from build123d import *

# Parameters (mm, degrees)
IZIM1_R                     = 7.95
Y_KSEKLIK_EKSTR_ZYON1_DEPTH = 8
IZIM2_R                     = 1.35
KES_EKSTR_ZYON1_DEPTH       = 50
IZIM3_R                     = 1.35
KES_EKSTR_ZYON2_DEPTH       = 29
KES_EKSTR_ZYON3_DEPTH       = 10
Y_KSEKLIK_EKSTR_ZYON2_REACH = 46.587
IZIM5_W                     = 5.529758539
IZIM5_H                     = 16.549351305
IZIM6_R                     = 1.35
KES_EKSTR_ZYON4_DEPTH       = 10
KES_EKSTR_ZYON5_DEPTH       = 2.5
Y_KSEKLIK_EKSTR_ZYON3_DEPTH = 0.5


with BuildPart() as part:
    # Çizim1 → Yükseklik-Ekstrüzyon1 (new body)
    with BuildSketch(Plane.XY):
        with BuildLine():
            Line((0, 0), (32, 0))
            Line((32, 0), (32, 8))
            Line((32, 8), (31.5, 8))
            ThreePointArc((31.5, 8), (28.671572875, 9.171572875), (27.5, 12))
            Line((27.5, 12), (27.5, 18))
            ThreePointArc((27.5, 18), (28.671572875, 20.828427125), (31.5, 22))
            Line((31.5, 22), (32, 22))
            Line((32, 22), (32, 30))
            Line((32, 30), (0, 30))
            Line((0, 30), (0, 22))
            Line((0, 22), (0.5, 22))
            ThreePointArc((0.5, 22), (3.328427125, 20.828427125), (4.5, 18))
            Line((4.5, 18), (4.5, 12))
            ThreePointArc((4.5, 12), (3.328427125, 9.171572875), (0.5, 8))
            Line((0.5, 8), (0, 8))
            Line((0, 8), (0, 0))
        make_face()
        with Locations((16, 15)):
            Circle(IZIM1_R, mode=Mode.SUBTRACT)
    extrude(amount=Y_KSEKLIK_EKSTR_ZYON1_DEPTH)

    # Çizim2 → Kes-Ekstrüzyon1 (cut)
    with BuildSketch(Plane(origin=(32, 0, 0), x_dir=(0, 0, -1), z_dir=(1, 0, 0))):
        with Locations((-4, 4)):
            Circle(IZIM2_R)
        with Locations((-4, 26)):
            Circle(IZIM2_R)
    extrude(amount=-KES_EKSTR_ZYON1_DEPTH, mode=Mode.SUBTRACT)

    # Çizim3 → Kes-Ekstrüzyon2 (cut)
    with BuildSketch(Plane.ZY.offset(-4.5)):
        with Locations(Location((4, 15, 0), (0, 0, 270))):
            Circle(IZIM3_R)
    extrude(amount=-KES_EKSTR_ZYON2_DEPTH, mode=Mode.SUBTRACT)

    # Çizim4 → Kes-Ekstrüzyon3 (cut)
    with BuildSketch(Plane(origin=(0, 0, 0), x_dir=(-1, 0, 0), z_dir=(0, 0, -1))):
        Polygon((-16, 30), (-16, 0), (9.241069926, -10.278514345), (11.843794838, 24.557008953), (11.843794838, 39.531622814), align=None)
    extrude(amount=-KES_EKSTR_ZYON3_DEPTH, mode=Mode.SUBTRACT)

    # Yükseklik-Ekstrüzyon2: up to this face of the body (flat: up to its plane)
    y_kseklik_ekstr_zyon2_end = Plane(part.part.faces().sort_by_distance((24.391799767, 15, 8))[0])
    # Çizim5 → Yükseklik-Ekstrüzyon2 (add, up to the picked face)
    with BuildSketch(Plane(origin=(0, 0, 0), x_dir=(-1, 0, 0), z_dir=(0, 0, -1)), mode=Mode.PRIVATE) as y_kseklik_ekstr_zyon2_sk1:
        with Locations((-29.235120731, 13.725324347)):
            Rectangle(IZIM5_W, IZIM5_H)
    y_kseklik_ekstr_zyon2_tool1 = split(extrude(y_kseklik_ekstr_zyon2_sk1.sketch, amount=-Y_KSEKLIK_EKSTR_ZYON2_REACH, mode=Mode.PRIVATE), bisect_by=y_kseklik_ekstr_zyon2_end, keep=Keep.BOTH, mode=Mode.PRIVATE)
    add(y_kseklik_ekstr_zyon2_tool1.solids().sort_by(Axis((29.235121, 13.725324, 0), (0, 0, 1)))[0])

    # Çizim6 → Kes-Ekstrüzyon4 (cut)
    with BuildSketch(Plane.ZY.offset(-26.470241461)):
        with Locations(Location((4, 15, 0), (0, 0, 270))):
            Circle(IZIM6_R)
    extrude(amount=-KES_EKSTR_ZYON4_DEPTH, mode=Mode.SUBTRACT)

    # Çizim7 → Kes-Ekstrüzyon5 (cut)
    with BuildSketch(Plane(origin=(32, 0, 0), x_dir=(0, 0, -1), z_dir=(1, 0, 0))):
        Polygon((-2.41228676, 28.75), (-5.58771324, 28.75), (-7.175426481, 26), (-5.58771324, 23.25), (-2.41228676, 23.25), (-0.824573519, 26), align=None)
        Polygon((-0.824573519, 15), (-2.41228676, 17.75), (-5.58771324, 17.75), (-7.175426481, 15), (-5.58771324, 12.25), (-2.41228676, 12.25), align=None)
        Polygon((-2.41228676, 6.75), (-5.58771324, 6.75), (-7.175426481, 4), (-5.58771324, 1.25), (-2.41228676, 1.25), (-0.824573519, 4), align=None)
    extrude(amount=-KES_EKSTR_ZYON5_DEPTH, mode=Mode.SUBTRACT)

    # Çizim8 → Yükseklik-Ekstrüzyon3 (add)
    with BuildSketch(Plane.XY.offset(8)):
        with BuildLine():
            Line((32, 30), (32, 0))
            Line((32, 0), (16, 0))
            Line((16, 0), (16, 7.05))
            ThreePointArc((16, 7.05), (23.95, 15), (16, 22.95))
            Line((16, 22.95), (16, 30))
            Line((16, 30), (32, 30))
        make_face()
    y_kseklik_ekstr_zyon3 = extrude(amount=Y_KSEKLIK_EKSTR_ZYON3_DEPTH)

    # Aynalama1: Yükseklik-Ekstrüzyon3 across plane
    add(y_kseklik_ekstr_zyon3.mirror(Plane.XY.offset(4)))


solid = part.part
The listing builds one solid part. Answer for the finished solid, in the listing's coordinates (mm). A direction names the side the tool comes from. Give positions to 0.01 mm unless a question says otherwise; leave off trailing zeros. Write each loop counter-clockwise with the first axis right and the second up, starting at its lowest first coordinate (ties: lowest second). Pieces come first, ordered by that corner, then holes. Notation, with made-up numbers: (-35.5, 69) - (4.5, 69) arc R19 cw to (4.5, 73) - close; hole circle Ø7 at (-14.75, -28). An arc over 180 degrees is marked (long way). One line per question, with ' | ' between items. Start each with the question number.
1. Section B-B, the plane x = 30.5 is taken. Determine the outline of the cut face in (y, z).
2. Determine the mould class of faces 3 (the face through (26, 15, 8.5)), 4 (the face through (32, 19, 4)), 5 (the face through (22.84, 2.8, 3.38)) for opening direction Z: +Z half, -Z half, draft (parallel to the pull), parting line (faces both ways), or undercut.
3. Section A-A, the plane x = 18 is taken. Determine the outline of the cut face in (y, z).
4. Section C-C, the plane z = 4.5 is taken. Count the separate pieces of the cut face and the enclosed holes in it, then the cut area to 3 significant figures.
5. Given P1, Ø1.6, axis at y = 14.5, z = 4, coming from the +X side; P2, Ø5, axis at y = 16.5, z = 1, coming from the -X side, each flat-ended and moving along its own axis, determine where each tip first touches the part or whether it passes through.
6. For faces 1 (the face through (31, 6.75, 4)), 2 (the face through (24, 0, 4)), determine the directions among +Z, -Z, +X, -X, +Y, -Y from which every point of the face is accessible in a straight line to the end or side of a thin tool.
7. Section D-D, the plane y = 23.75 is taken. Determine the outline of the cut face in (x, z), then the cut area to 3 significant figures.
8. Straight lines are drawn through the part: line 1 (Y direction, x = 28, z = 4); line 2 (Y direction, x = 30, z = 4); line 3 (Z direction, x = 23, y = 25.75). For each, find the intervals that lie inside material, in ascending order.
Result:
1) outline: (0, -0.5) - (30, -0.5) - (30, 8.5) - (0, 8.5) - close; hole (1.25, 2.41) - (4, 0.82) - (6.75, 2.41) - (6.75, 5.59) - (4, 7.18) - (1.25, 5.59) - close; hole (12.25, 2.41) - (15, 0.82) - (17.75, 2.41) - (17.75, 5.59) - (15, 7.18) - (12.25, 5.59) - close; hole (23.25, 2.41) - (26, 0.82) - (28.75, 2.41) - (28.75, 5.59) - (26, 7.18) - (23.25, 5.59) - close
2) face 3: +Z half | face 4: draft | face 5: undercut
3) outline: (0, -0.5) - (7.31, -0.5) - (7.31, 8.5) - (0, 8.5) - close; (22.69, -0.5) - (30, -0.5) - (30, 8.5) - (22.69, 8.5) - close; hole circle Ø2.7 at (4, 4); hole circle Ø2.7 at (26, 4)
4) separate pieces: 4 | enclosed holes: 0 | area: 258 mm2
5) P1: passes through | P2: stops at x = 22.87
6) face 1: +X | face 2: +Z, -Z, +X, -X, -Y
7) outline: (16, -0.5) - (32, -0.5) - (32, 2.12) - (29.5, 2.12) - (29.5, 5.88) - (32, 5.88) - (32, 8.5) - (16, 8.5) - close | area: 135 mm2
8) line 1: y = 0 to 2.65, 5.35 to 13.65, 16.35 to 24.65, 27.35 to 30 | line 2: y = 0 to 1.25, 6.75 to 12.25, 17.75 to 23.25, 28.75 to 30 | line 3: z = -0.5 to 2.67, 5.33 to 8.5
